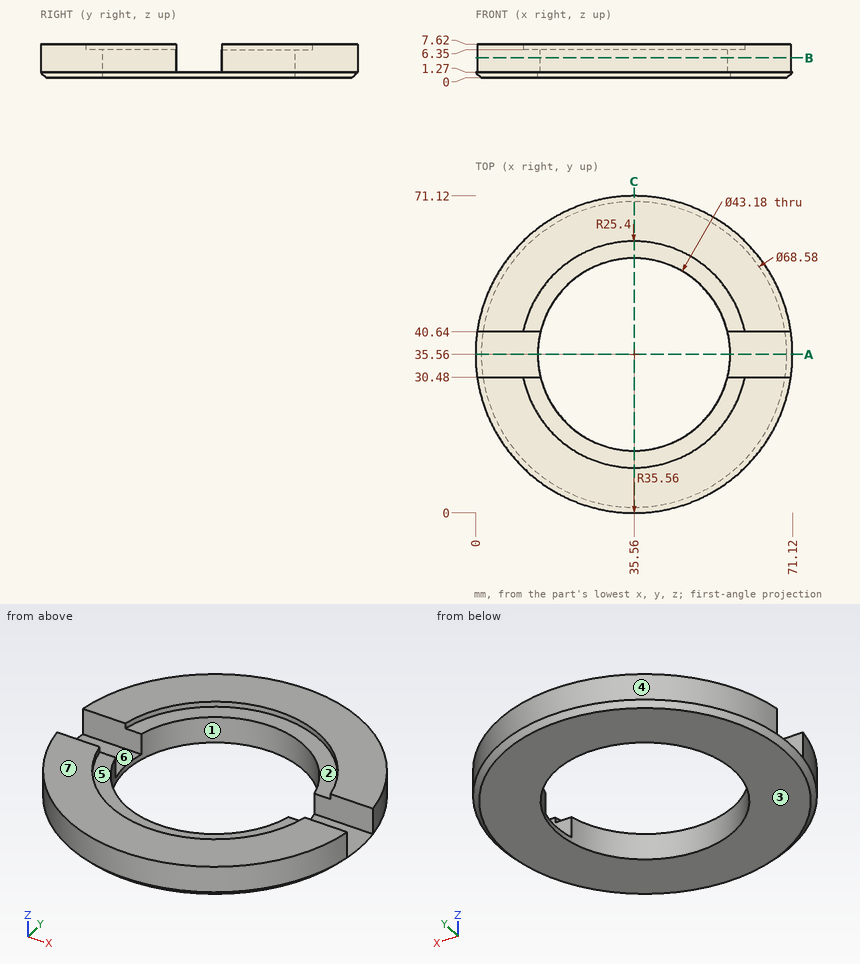
Input: dimensioned drawing with shaded views. Units: mm. Origin: part minimum x, y, z. A direction names the side the tool comes from. Coordinates: 2 decimals unless noted, no trailing zeros. Order: outer loops, then holes, each group sorted by start corner. A loop starts at its lowest first (then second) coordinate and runs counter-clockwise, first axis right, second up. Notation, with made-up numbers: (86, 80.5) - (117, 80.5) arc R29 ccw to (117, 119.5) - close; hole circle Ø8 at (-39.5, 56.5). An arc over 180 degrees is marked (long way). One line per item, written item: value.
1) Mould query, pull axis X, two halves, no side actions, for the marked faces 1, 2, 3 and 4. Classes: released by +X, released by -X, zero draft, split by the parting line, or undercut.
Computed values:
face 1: undercut
face 2: undercut
face 3: zero draft
face 4: split by the parting line
2) Reachability of the marked faces 5, 6 and 7 from +Z, -Z, +X, -X, +Y, -Y: full face, straight path, thin tool, end or side. Return the list, or none.
Computed values:
face 5: +Z
face 6: +Z, +X, -X
face 7: +Z, +X, -X, +Y, -Y
3) Cut plane A-A on y = 35.56. Output: boundary loops of the cut face in (x, z).
Computed values:
outline: (0, 1.27) - (1.27, 0) - (13.97, 0) - (13.97, 1.27) - close; (57.15, 0) - (69.85, 0) - (71.12, 1.27) - (57.15, 1.27) - close
4) Cut plane C-C on x = 35.56. Output: boundary loops of the cut face in (y, z), plus the area to 3 significant figures.
Computed values:
outline: (0, 1.27) - (1.27, 0) - (13.97, 0) - (13.97, 6.35) - (10.16, 6.35) - (10.16, 7.62) - (0, 7.62) - close; (57.15, 0) - (69.85, 0) - (71.12, 1.27) - (71.12, 7.62) - (60.96, 7.62) - (60.96, 6.35) - (57.15, 6.35) - close
area: 202 mm^2
5) Ray query, line 1 (Y direction, x = 35.56, z = 2.5); line 2 (Z direction, x = 61, y = 31); line 3 (Y direction, x = 20, z = 1). Return the intervals inside material, ascending. Write a range as [from, to].
Computed values:
line 1: y = [0, 13.97], [57.15, 71.12]
line 2: z = [0, 1.27]
line 3: y = [3.89, 20.59], [50.53, 67.23]
6) Cut plane B-B on z = 4.5. Output: boundary loops of the cut face in (x, y).
Computed values:
outline: (0.36, 30.48) arc R35.56 ccw to (70.76, 30.48) - (56.54, 30.48) arc R21.59 cw to (14.58, 30.48) - close; (0.36, 40.64) - (14.58, 40.64) arc R21.59 cw to (56.54, 40.64) - (70.76, 40.64) arc R35.56 ccw to start
7) Contact query for flat-ended pins moving along their axis: pin 1 (2 mm diameter, centred on x = 19, z = 2.5, fed in from +Y) (3 decimals); pin 2 (2 mm diameter, centred on x = 43, z = 4.5, fed in from -Y); pin 3 (4 mm diameter, centred on x = 43, y = 16, fed in from +Z). Output: stop coordinate, or through.
Computed values:
pin 1: stops at y = 67.535
pin 2: stops at y = 0.59
pin 3: stops at z = 6.35
